Part model, mm, in its own coordinate system. Face numbers are marked on the shaded views. A direction names the side the tool comes from. Coordinates: 2 decimals unless noted, no trailing zeros. Loops run counter-clockwise (first coordinate to the right, second up) from the corner with the lowest first, then second, coordinate; pieces in that order, holes last. Notation, with made-up numbers: (-34.5, -10.75) -> (15.5, -10.75) arc R32 cw to (15.5, 21.25) -> close; hole circle Ø11 at (-3, -24.75). An arc over 180 degrees is marked (long way). One line per question, with ' | ' between items. Start each with the question number.
1) Cut at B-B (z = 8). List the corners of the cut face in (x, y) (3 decimals), plus the area to 3 significant figures.
2) Probe L1, parallel to X at y = 0, z = 9.5 (3 decimals); L2, parallel to X at y = 0, z = -3; L3, parallel to Z at x = 0.25, y = -10. List the from-to ranges inside material, lowest first. Write a range as from..to.
3) Cut at A-A (z = -7.5). List the corners of the cut face in (x, y), plus the area to 3 significant figures.
4) 3-axis set-ups, long thin cutter, end or side, ignore diameter. For the marked faces 5, 6 and 7: which of +Z, -Z, +X, -X, +Y, -Y reach the whole face in a straight line?
5) Drop flat-ended pins along their axis: pin 1 (6.5 mm diameter, centred on x = 0, y = 0, fed in from -Z); pin 2 (1.5 mm diameter, centred on x = -6, z = -15, fed in from +Y); pin 3 (1.5 mm diameter, centred on y = -6, z = -11, fed in from +X); pin 4 (1 mm diameter, centred on y = -8, z = -4.5, fed in from -X). Give the stop position or say it passes through.
6) Two-plate mould, pull along Z, no slides. Class the marked faces 1, 2, 3 and 4: released by +Z, released by -Z, zero draft, split by the parting line, or undercut.
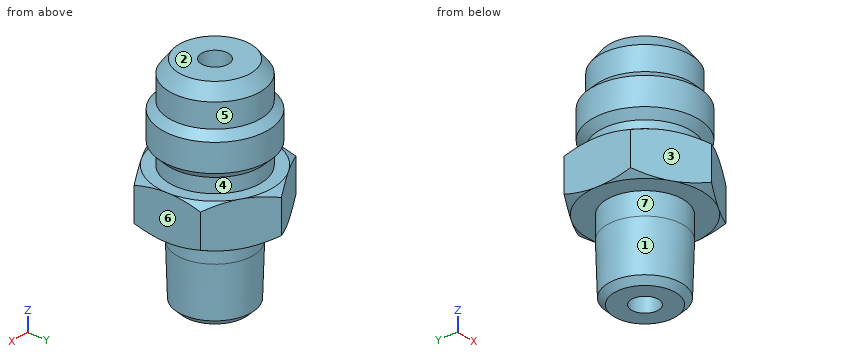
from build123d import *

# Parameters (mm, degrees)
SKETCH2_R           = 10.19175
BOSS_EXTRUDE1_DEPTH = 7.874


with BuildPart() as part:
    # Sketch1 → Revolve1 (revolve)
    with BuildSketch(Plane(origin=(0, 0, 0), x_dir=(0, 0, -1), z_dir=(1, 0, 0))):
        Polygon((-19.446875, 2.413), (-19.446875, 6.448056668), (-17.138253125, 8.187728032), (-12.8508125, 8.187728032), (-11.513540532, 9.525), (-6.568084468, 9.525), (-5.2308125, 8.187728032), (-2.651125, 8.187728032), (-2.651125, 10.31875), (5.222875, 10.31875), (5.222875, 6.858), (9.241155, 6.858), (18.354531448, 6.574254175), (19.446875, 5.481910623), (19.446875, 2.413), align=None)
    revolve(axis=Axis((0, 0, 19.446875), (0, 0, -1)))

    # Sketch2 → Boss-Extrude1 (add)
    with BuildSketch(Plane.XY.offset(2.651125)):
        Polygon((0, 11.91506618), (-10.31875, 5.95753309), (-10.31875, -5.95753309), (0, -11.91506618), (10.31875, -5.95753309), (10.31875, 5.95753309), align=None)
        Circle(SKETCH2_R, mode=Mode.SUBTRACT)
    extrude(amount=-BOSS_EXTRUDE1_DEPTH)

    # Sketch3 → Cut-Revolve1 (revolve, cut)
    with BuildSketch(Plane(origin=(0, 0, 0), x_dir=(0, 0, -1), z_dir=(1, 0, 0))):
        Polygon((-2.651125, 10.31875), (-2.651125, 11.91506618), (-1.729491424, 11.91506618), align=None)
        Polygon((4.301241424, 11.91506618), (5.222875, 10.31875), (5.222875, 11.91506618), align=None)
    revolve(axis=Axis((0, 0, 19.446875), (0, 0, -1)), mode=Mode.SUBTRACT)


solid = part.part
Reported:
1) outline: circle Ø19.05 at (0, 0); hole circle Ø4.826 at (0, 0) | area: 267 mm²
2) L1: x = -9.525..-2.413, 2.413..9.525 | L2: x = -10.32..-2.41, 2.41..10.32 | L3: z = -5.22..2.65
3) outline: circle Ø13.72 at (0, 0); hole circle Ø4.83 at (0, 0) | area: 129 mm²
4) face 5: +Z | face 6: +Z, -Z, +X, +Y, -Y | face 7: -Z
5) pin 1: stops at z = -19.45 | pin 2: stops at y = 4.13 | pin 3: stops at x = 4.33 | pin 4: stops at x = -7.65
6) face 1: released by -Z | face 2: released by +Z | face 3: zero draft | face 4: undercut
